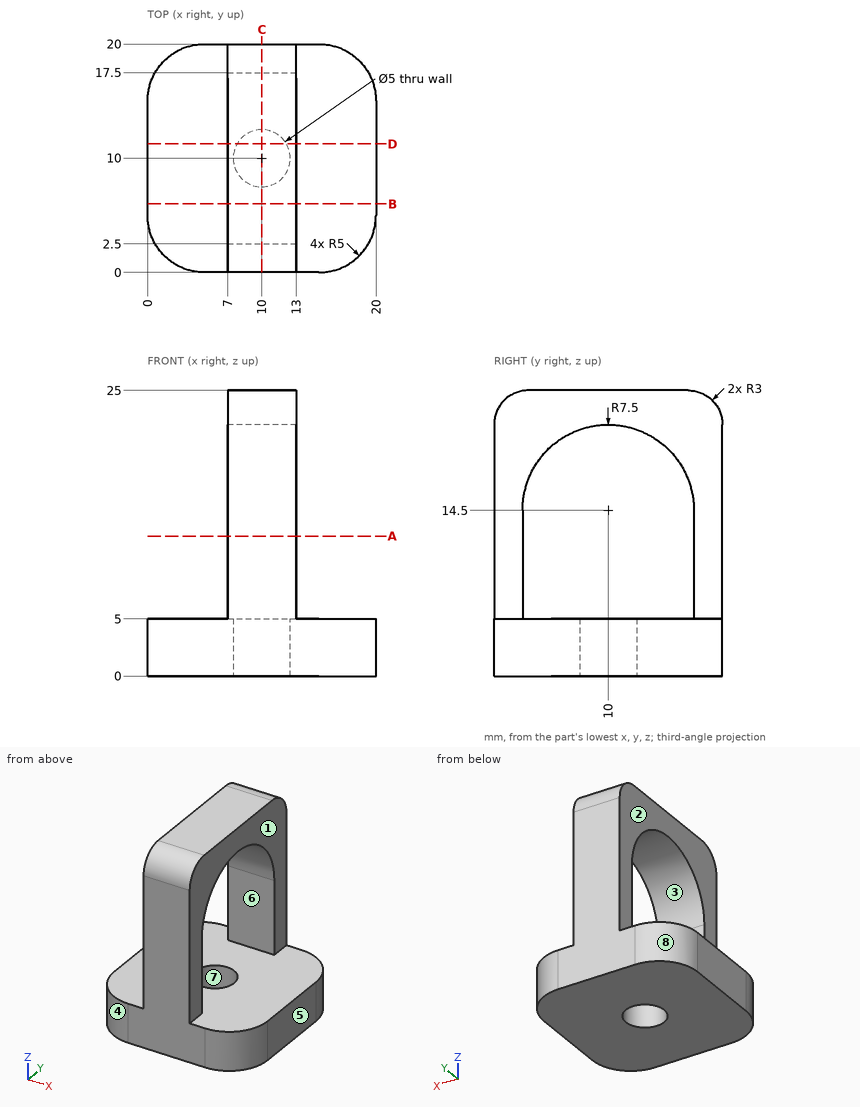
Can you work these out from the drawing? Everything is in mm from the part's minimum corner. A direction names the side the tool comes from. Round coordinates to 2 decimals unless told otherwise and drop trailing zeros. Loops run counter-clockwise (first coordinate to the right, second up) from the corner with the lowest first, then second, coordinate; pieces in that order, holes last. Notation, with made-up numbers: (13.25, 34.25) - (34.25, 34.25) arc R11 ccw to (34.25, 49.25) - close; hole circle Ø10 at (-36, 66). An arc over 180 degrees is marked (long way). Write item = value, one per line. Start each with the question number.
(1) If we section it at A-A (z = 12.25): Please give me the cut outline in (x, y).
(2) If we section it at B-B (y = 6): Please give me the cut outline in (x, z).
(3) If I drill on probe 1 along Y at (x, z) = (10.25, 5.75); probe 2 along Z at (x, y) = (2.5, 3.75); probe 3 along Y at (x, z) = (10, 2), over which ranges is the centre line in solid material (lowest first)? Write a range as [from, to].
(4) If we mould it in two halves opening along Y, with no side actions, what happens to the marked faces 5, 6, 7 and 8? For each: released by +Y, released by -Y, zero draft, split by the parting line, or undercut.
(5) For the marked faces 1, 2, 3 and 4, which set-ups out of +Z, -Z, +X, -X, +Y, -Y let a thin tool reach every point of the face, with its end or its side?
(6) If we section it at C-C (x = 10): Please give me the cut outline in (y, z).
(7) If we section it at D-D (y = 11.25): Please give me the cut outline in (x, z), and give its area (3 significant figures).
(8) For P1, Ø4, axis at x = 17.5, y = 3, coming from the +Z side; P2, Ø6, axis at y = 8, z = 14, coming from the +X side; P3, Ø10, axis at y = 6, z = 13, coming from the -X side, each with a flat end and sliding along its axis, tell me the tip position at first contact or that it passes through.
Ans:
q1.outline = (7, 0) - (13, 0) - (13, 2.5) - (7, 2.5) - close; (7, 17.5) - (13, 17.5) - (13, 20) - (7, 20) - close
q2.outline = (0, 0) - (20, 0) - (20, 5) - (0, 5) - close; (7, 20.84) - (13, 20.84) - (13, 25) - (7, 25) - close
q3.probe_1 = [0, 2.5], [17.5, 20]
q3.probe_2 = [0, 5]
q3.probe_3 = [0, 7.5], [12.5, 20]
q4.face_5 = zero draft
q4.face_6 = undercut
q4.face_7 = undercut
q4.face_8 = released by +Y
q5.face_1 = +Z, +X, +Y, -Y
q5.face_2 = +Z, -X, +Y, -Y
q5.face_3 = +X, -X
q5.face_4 = +Z, -Z, -X, -Y
q6.outline = (0, 0) - (7.5, 0) - (7.5, 5) - (2.5, 5) - (2.5, 14.5) arc R7.5 cw to (17.5, 14.5) - (17.5, 5) - (12.5, 5) - (12.5, 0) - (20, 0) - (20, 22) arc R3 ccw to (17, 25) - (3, 25) arc R3 ccw to (0, 22) - close
q7.outline = (0, 0) - (7.83, 0) - (7.83, 5) - (0, 5) - close; (7, 21.9) - (13, 21.9) - (13, 25) - (7, 25) - close; (12.17, 0) - (20, 0) - (20, 5) - (12.17, 5) - close
q7.area = 97.0 mm²
q8.P1 = 5
q8.P2 = through
q8.P3 = 7
